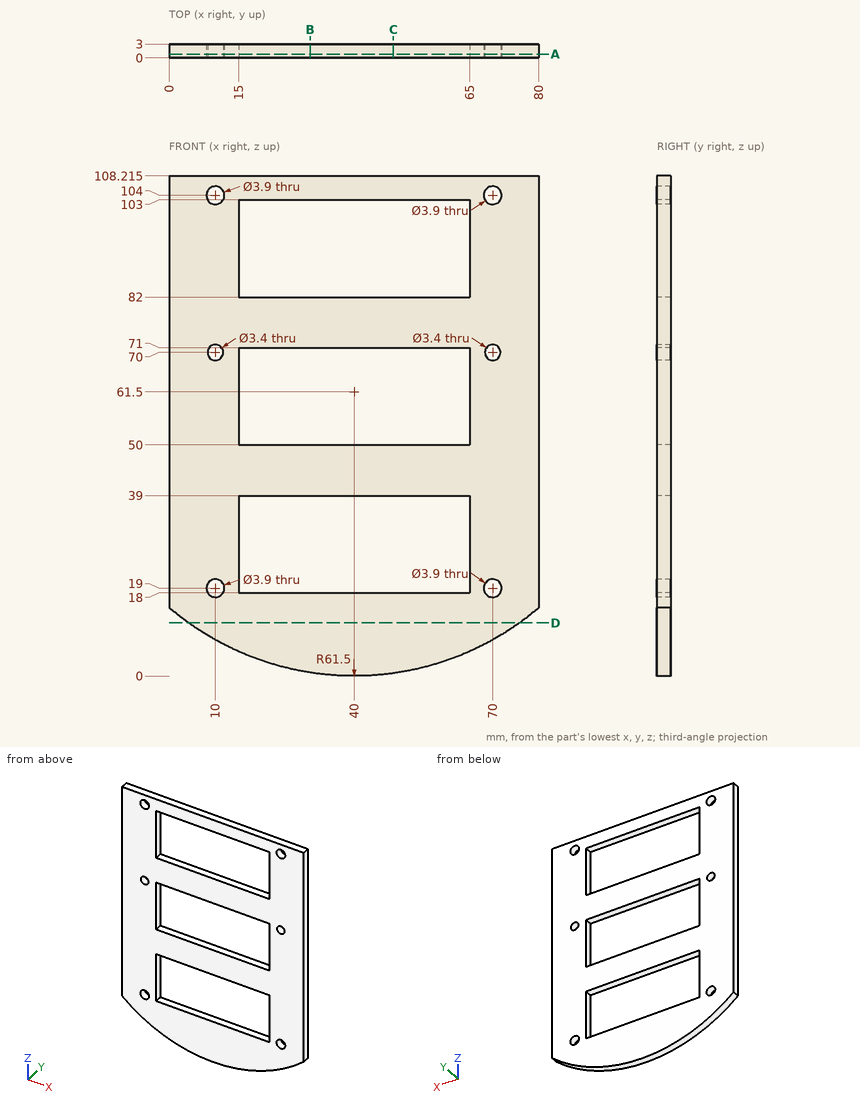
Input: dimensioned drawing with shaded views. Units: mm. Origin: part minimum x, y, z. Coordinates: 2 decimals unless noted, no trailing zeros. Order: outer loops, then holes, each group sorted by start corner. A loop starts at its lowest first (then second) coordinate and runs counter-clockwise, first axis right, second up. Notation, with made-up numbers: (64, -11.75) - (105, -11.75) arc R31 ccw to (105, 23.25) - close; hole circle Ø10 at (-8, 34). An arc over 180 degrees is marked (long way). Put each result on its own line as item: value.
1. Line query: line 1 along X through (y, z) = (2.15, 70); line 2 along X through (y, z) = (1.4, 104); line 3 along X through (y, z) = (1.05, 19). Output: solid intervals per line, ascending.
Report:
line 1: x = 0 to 8.3, 11.7 to 15, 65 to 68.3, 71.7 to 80
line 2: x = 0 to 8.05, 11.95 to 68.05, 71.95 to 80
line 3: x = 0 to 8.05, 11.95 to 15, 65 to 68.05, 71.95 to 80
2. Cut plane A-A on y = 0.8. State how many separate pieces and enclosed holes the cut face has, then the cut area to 3 significant figures.
Report:
separate pieces: 1
enclosed holes: 9
area: 5,070 mm2
3. Contact query for flat-ended pins moving along their axis: pin 1 Ø3 at (x, z) = (10, 70) entering from -Y; pin 2 Ø0.9 at (x, y) = (42.5, 1) entering from -Z; pin 3 Ø0.9 at (x, y) = (30, 1) entering from -Z. Output: stop coordinate, or through.
Report:
pin 1: passes through
pin 2: stops at z = 0.03
pin 3: stops at z = 0.75
4. Cut plane C-C on x = 48.5. Return the cut outline in (y, z) (1 decimal).
Report:
outline: (0, 0.6) - (3, 0.6) - (3, 18) - (0, 18) - close; (0, 39) - (3, 39) - (3, 50) - (0, 50) - close; (0, 71) - (3, 71) - (3, 82) - (0, 82) - close; (0, 103) - (3, 103) - (3, 108.2) - (0, 108.2) - close
5. Cut plane B-B on x = 30.5. Return the cut outline in (y, z) (1 decimal).
Report:
outline: (0, 0.7) - (3, 0.7) - (3, 18) - (0, 18) - close; (0, 39) - (3, 39) - (3, 50) - (0, 50) - close; (0, 71) - (3, 71) - (3, 82) - (0, 82) - close; (0, 103) - (3, 103) - (3, 108.2) - (0, 108.2) - close
6. Cut plane D-D on z = 11.5. Return the cut outline in (x, y).
Report:
outline: (4.19, 0) - (75.81, 0) - (75.81, 3) - (4.19, 3) - close
